The listing builds one solid part. Answer for the finished solid, in the listing's coordinates (mm). A direction names the side the tool comes from. Give positions to 0.01 mm unless a question says otherwise; leave off trailing zeros. Loops run counter-clockwise (first coordinate to the right, second up) from the corner with the lowest first, then second, coordinate; pieces in that order, holes last. Notation, with made-up numbers: (38, 60) - (78, 60) arc R6 ccw to (78, 65) - close; hole circle Ø9 at (12, 72.25). An arc over 180 degrees is marked (long way). Write item = value, one per line. Start each with the question number.
1) The part is cut by section D-D on y = 0. Write down the section's boundary in (x, z).
2) Flat-ended cylindrical pins translate along their axes: P1, Ø5.5, axis at x = 15, y = 15, coming from the +Z side; P2, Ø8.5, axis at x = 30, y = 25, coming from the -Z side; P3, Ø7, axis at x = 17, y = -15, coming from the +Z side. Find the tip coordinate at first contact, or state that the pin passes through.
3) Consider probe 1 along Y at (x, z) = (-5, 12.75); probe 2 along Y at (x, z) = (15, 1.9); probe 3 along X at (y, z) = (17, 2.5). Determine where each line is inside the solid, lowest interval first.
4) The part is cut by section A-A on y = -25. Write down the section's boundary in (x, z), plus the area to 3 significant figures.
5) The part is cut by section C-C on x = 4. Write down the section's boundary in (y, z).
6) The mould has two halves that part along Y. Classify faces 5 (the flat face through (-1, 25, 20)), 6 (the cylindrical face through (-30.338, 27.578, 12.753)): +Y half, -Y half, draft (parallel to the pull), parting line (faces both ways), or undercut.
7) The part is cut by section B-B on z = 8. State how many separate pieces and enclosed holes the cut face has, plus the area to 3 significant figures.
8) Which of the six approach directions +Z, -Z, +X, -X, +Y, -Y give full straight-line access (tool end or side, diameter ignored) to faces 1 (the flat face through (-1, 0, 10)), 2 (the flat face through (17, -17, 4)), 3 (the flat face through (-32, -27, 5.3)), 4 (the cylindrical face through (-17.4, -16, 2))?
from build123d import *

# Parameters (mm, degrees)
SKIZZE1_W                       = 80
SKIZZE1_H                       = 60
AUFSATZ_LINEAR_AUSTRAGEN1_DEPTH = 10
SKIZZE2_W                       = 80
SKIZZE2_H                       = 10
AUFSATZ_LINEAR_AUSTRAGEN2_DEPTH = 10
SKIZZE5_R                       = 2.6
SCHNITT_LINEAR_AUSTRAGEN3_DEPTH = 20
SKIZZE6_R                       = 11
SCHNITT_LINEAR_AUSTRAGEN4_DEPTH = 12.2
FASE1_SIZE                      = 1
SKIZZE7_R                       = 4.5
SCHNITT_LINEAR_AUSTRAGEN5_DEPTH = 5.3
SKIZZE8_R                       = 2.6
SCHNITT_LINEAR_AUSTRAGEN6_DEPTH = 10
SKIZZE9_R                       = 4.5
SCHNITT_LINEAR_AUSTRAGEN7_DEPTH = 6


with BuildPart() as part:
    # Skizze1 → Aufsatz-Linear austragen1 (new body)
    with BuildSketch(Plane.XY):
        Rectangle(SKIZZE1_W, SKIZZE1_H)
    extrude(amount=AUFSATZ_LINEAR_AUSTRAGEN1_DEPTH)

    # Skizze2 → Aufsatz-Linear austragen2 (add)
    with BuildSketch(Plane.XY.offset(10)):
        with Locations((0, 25)):
            Rectangle(SKIZZE2_W, SKIZZE2_H)
        with Locations((0, -25)):
            Rectangle(SKIZZE2_W, SKIZZE2_H)
    extrude(amount=AUFSATZ_LINEAR_AUSTRAGEN2_DEPTH)

    # Skizze5 → Schnitt-Linear austragen3 (cut)
    with BuildSketch(Plane.XY.offset(20)):
        with Locations((30, 25)):
            Circle(SKIZZE5_R)
        with Locations((-30, 25)):
            Circle(SKIZZE5_R)
        with Locations((-30, -25)):
            Circle(SKIZZE5_R)
        with Locations((30, -25)):
            Circle(SKIZZE5_R)
    extrude(amount=-SCHNITT_LINEAR_AUSTRAGEN3_DEPTH, mode=Mode.SUBTRACT)

    # Skizze6 → Schnitt-Linear austragen4 (cut)
    with BuildSketch(Plane.XY.offset(10)):
        with Locations((-25, 0)):
            Circle(SKIZZE6_R)
        with Locations((25, 0)):
            Circle(SKIZZE6_R)
    extrude(amount=-SCHNITT_LINEAR_AUSTRAGEN4_DEPTH, mode=Mode.SUBTRACT)

    # Fase1
    fase1_edges = [part.edges().sort_by_distance(p)[0] for p in [
        (-36, 0, 0),
        (14, 0, 0),
    ]]
    chamfer(fase1_edges, length=FASE1_SIZE)

    # Skizze7 → Schnitt-Linear austragen5 (cut)
    with BuildSketch(Plane(origin=(0, 0, 0), x_dir=(-1, 0, 0), z_dir=(0, 0, -1))):
        with Locations((-30, 25)):
            Circle(SKIZZE7_R)
        with Locations((30, 25)):
            Circle(SKIZZE7_R)
        with Locations((30, -25)):
            Circle(SKIZZE7_R)
        with Locations((-30, -25)):
            Circle(SKIZZE7_R)
    extrude(amount=-SCHNITT_LINEAR_AUSTRAGEN5_DEPTH, mode=Mode.SUBTRACT)

    # Skizze8 → Schnitt-Linear austragen6 (cut)
    with BuildSketch(Plane(origin=(0, 0, 0), x_dir=(-1, 0, 0), z_dir=(0, 0, -1))):
        with Locations((-15, 15)):
            Circle(SKIZZE8_R)
        with Locations((15, 15)):
            Circle(SKIZZE8_R)
        with Locations((15, -15)):
            Circle(SKIZZE8_R)
        with Locations((-15, -15)):
            Circle(SKIZZE8_R)
    extrude(amount=-SCHNITT_LINEAR_AUSTRAGEN6_DEPTH, mode=Mode.SUBTRACT)

    # Skizze9 → Schnitt-Linear austragen7 (cut)
    with BuildSketch(Plane.XY.offset(10)):
        with Locations((15, 15)):
            Circle(SKIZZE9_R)
        with Locations((-15, 15)):
            Circle(SKIZZE9_R)
        with Locations((-15, -15)):
            Circle(SKIZZE9_R)
        with Locations((15, -15)):
            Circle(SKIZZE9_R)
    extrude(amount=-SCHNITT_LINEAR_AUSTRAGEN7_DEPTH, mode=Mode.SUBTRACT)


solid = part.part
Answer below:
q1.outline = (-40, 0) - (-37, 0) - (-36, 1) - (-36, 10) - (-40, 10) - close; (-14, 1) - (-13, 0) - (13, 0) - (14, 1) - (14, 10) - (-14, 10) - close; (36, 1) - (37, 0) - (40, 0) - (40, 10) - (36, 10) - close
q2.P1 = 4
q2.P2 = 5.3
q2.P3 = 10
q3.probe_1 = -30 to -20, 20 to 30
q3.probe_2 = -30 to -17.6, -12.4 to -4.58, 4.58 to 12.4, 17.6 to 30
q3.probe_3 = -40 to -16.66, -13.34 to 13.34, 16.66 to 40
q4.outline = (-40, 0) - (-34.5, 0) - (-34.5, 5.3) - (-32.6, 5.3) - (-32.6, 20) - (-40, 20) - close; (-27.4, 5.3) - (-25.5, 5.3) - (-25.5, 0) - (25.5, 0) - (25.5, 5.3) - (27.4, 5.3) - (27.4, 20) - (-27.4, 20) - close; (32.6, 5.3) - (34.5, 5.3) - (34.5, 0) - (40, 0) - (40, 20) - (32.6, 20) - close
q4.area = 1,350 mm2
q5.outline = (-30, 0) - (30, 0) - (30, 20) - (20, 20) - (20, 10) - (-20, 10) - (-20, 20) - (-30, 20) - close
q6.face_5 = draft
q6.face_6 = undercut
q7.separate_pieces = 1
q7.enclosed_holes = 10
q7.area = 3,700 mm2
q8.face_1 = +Z, +X, -X
q8.face_2 = +Z
q8.face_3 = -Z
q8.face_4 = +Z, -Z
